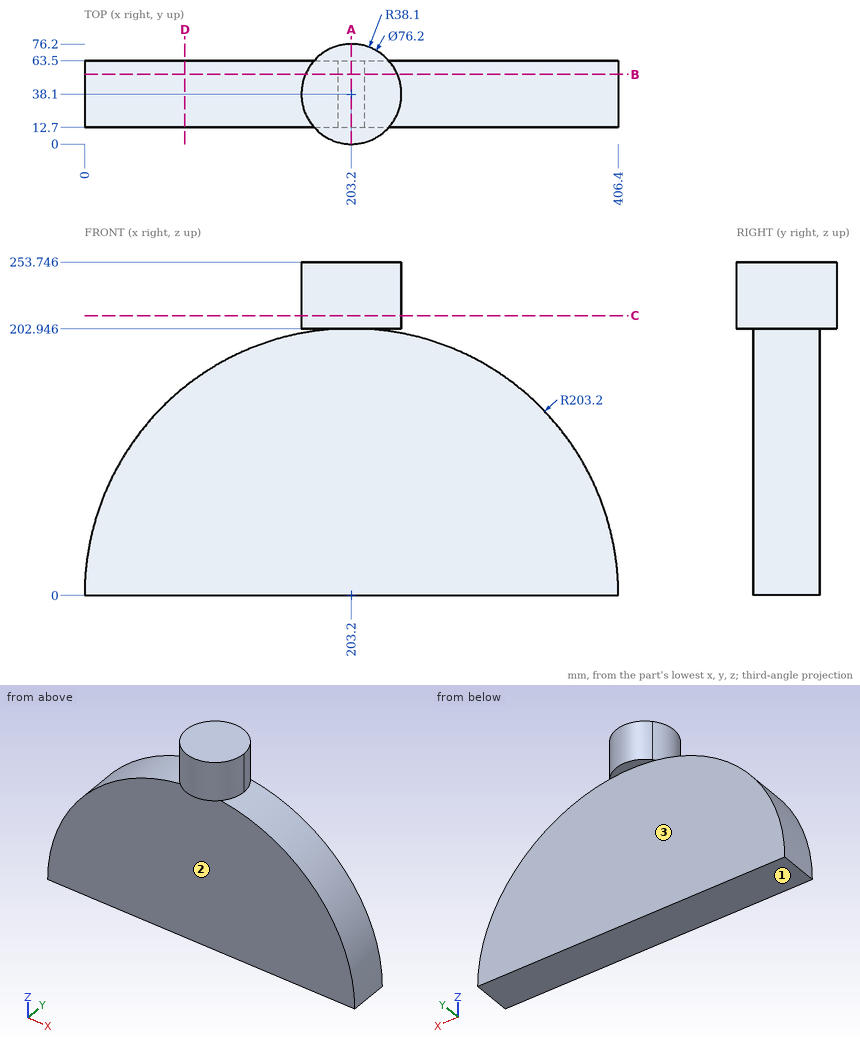
Drawing for the job (mm, zero at the part's lowest x, y, z). A direction names the side the tool comes from. Coordinates: 2 decimals unless noted, no trailing zeros. Order: outer loops, then holes, each group sorted by start corner. A loop starts at its lowest first (then second) coordinate and runs counter-clockwise, first axis right, second up. Notation, with made-up numbers: (47.5, 23.25) -> (102.5, 23.25) arc R17 cw to (102.5, 33.25) -> close; hole circle Ø7 at (-14, 55.25). An arc over 180 degrees is marked (long way). Answer in a Markdown table with one row per item.
1) Flat gauge pins, fed straight in: P1, Ø6, axis at y = 20.5, z = 89, coming from the -X side; P2, Ø5, axis at y = 14.5, z = 150, coming from the -X side; P3, Ø12, axis at y = 28, z = 206, coming from the +X side. Where does each tip first touch, or does it go through?
Check values:
| item | result |
|---|---|
| P1 | x = 19.1 |
| P2 | x = 63.44 |
| P3 | x = 241.08 |
2) Drill centre lines: line 1 (Y direction, x = 236.5, z = 129.5); line 2 (Z direction, x = 152, y = 24); line 3 (Z direction, x = 136.5, y = 20.5). Where is each one in solid material? Low to high.
Check values:
| item | result |
|---|---|
| line 1 | 12.7 to 63.5 |
| line 2 | 0 to 196.64 |
| line 3 | 0 to 191.94 |
3) Band-saw the part on C-C (z = 213). List the corners of the cut face in (x, y).
Check values:
| item | result |
|---|---|
| outline | circle Ø76.2 at (203.2, 38.1) |
4) Band-saw the part on D-D (x = 76.5). List the corners of the cut face in (y, z), and give its area (3 significant figures).
Check values:
| item | result |
|---|---|
| outline | (12.7, 0) -> (63.5, 0) -> (63.5, 158.86) -> (12.7, 158.86) -> close |
| area | 8,070 mm2 |
5) Band-saw the part on A-A (x = 203.2). List the corners of the cut face in (y, z).
Check values:
| item | result |
|---|---|
| outline | (0, 202.95) -> (12.7, 202.95) -> (12.7, 0) -> (63.5, 0) -> (63.5, 202.95) -> (76.2, 202.95) -> (76.2, 253.75) -> (0, 253.75) -> close |
6) Band-saw the part on B-B (y = 53). List the corners of the cut face in (x, z), and give its area (3 significant figures).
Check values:
| item | result |
|---|---|
| outline | (0, 0) -> (406.4, 0) arc R203.2 ccw to (213.36, 202.95) -> (238.27, 202.95) -> (238.27, 253.75) -> (168.13, 253.75) -> (168.13, 202.95) -> (193.04, 202.95) arc R203.2 ccw to start |
| area | 68,400 mm2 |
7) Which spindle directions (+Z, -Z, +X, -X, +Y, -Y) get a long thin tool onto all of the face, cutting with end or side? Do the marked faces 1, 2 and 3. Say none if no direction does.
Check values:
| item | result |
|---|---|
| face 1 | -Z, +X, -X, +Y, -Y |
| face 2 | -Z, +X, -X, -Y |
| face 3 | -Z, +X, -X, +Y |
